Here's how the part is built. I have some questions about the finished solid (model axes, mm). Face numbers are marked on the shaded views. A direction names the side the tool comes from. Give positions to 0.01 mm unless a question says otherwise; leave off trailing zeros. Loops run counter-clockwise (first coordinate to the right, second up) from the corner with the lowest first, then second, coordinate; pieces in that order, holes last.
Q1. For the marked faces 1 and 2, which set-ups out of +Z, -Z, +X, -X, +Y, -Y let a thin tool reach every point of the face, with its end or its side?
Q2. I need wall thicknesses on probe 1 along Z at (x, y) = (6.25, 0.05); probe 2 along Z at (x, y) = (1, 0.6); probe 3 along Z at (x, y) = (3.5, 0.55). Which ranges of each line are inside material? Lowest first, please.
Q3. Suppose I cut it at A-A (x = 6). List the corners of the cut face in (y, z) for me.
Q4. I'm going to push a flat-ended pin straight in: P1, Ø1, axis at x = 3, z = 1, coming from the +Y side. Where does the tip first touch, or does it pass through?
```python
from build123d import *

# Parameters (mm, degrees)
RECPAT_COUNT = 2
RECPAT_ANGLE = 90


with BuildPart() as part:
    # Fillet1: read off the stored shape, not the designer's step
    # Fillet1 outline → Fillet1 (revolve)
    with BuildSketch(Plane.YX):
        with BuildLine():
            Line((1.25, 2.2), (1.25, 7.1))
            Line((1.25, 7.1), (0, 7.1))
            Line((0, 7.1), (0, 0))
            ThreePointArc((0, 0), (1.267435139, 0.206109099), (2.404255321, 0.803195916))
            ThreePointArc((2.404255321, 0.803195916), (2.474733878, 0.88781572), (2.5, 0.99500416))
            Line((2.5, 0.99500416), (2.5, 2.1))
            Line((2.5, 2.1), (1.35, 2.1))
            ThreePointArc((1.35, 2.1), (1.279289322, 2.129289322), (1.25, 2.2))
        make_face()
    revolve(axis=Axis((0, 0, 0), (1, 0, 0)))

    # Sketch3 → Recess section 0
    with BuildSketch(Plane(origin=(0, 0, 0), x_dir=(0, 0, -1), z_dir=(1, 0, 0))):
        with BuildLine():
            Line((0.37, -1.3), (-0.37, -1.3))
            Line((-0.37, -1.3), (-0.37, 1.3))
            Line((-0.37, 1.3), (0.37, 1.3))
            Line((0.37, 1.3), (0.37, -1.3))
        make_face()
    # Sketch4 → Recess section 1
    with BuildSketch(Plane(origin=(1.5, 0, 0), x_dir=(0, 0, -1), z_dir=(1, 0, 0))):
        with BuildLine():
            Line((0.37, -0.552127713), (-0.37, -0.552127713))
            Line((-0.37, -0.552127713), (-0.37, 0.552127713))
            Line((-0.37, 0.552127713), (0.37, 0.552127713))
            Line((0.37, 0.552127713), (0.37, -0.552127713))
        make_face()
    recess = loft(mode=Mode.SUBTRACT)

    # RecPat: Recess ×2 about axis
    recpat_axis = Axis((0, 0, 0), (1, 0, 0))
    for i in range(1, RECPAT_COUNT):
        add(recess.rotate(recpat_axis, i * RECPAT_ANGLE / (RECPAT_COUNT - 1)), mode=Mode.SUBTRACT)

    # RecCorSke → RecessCore (revolve, cut)
    with BuildSketch(Plane.XY, mode=Mode.PRIVATE) as recesscore_sk:
        Polygon((0, 0), (0, 0.660890218), (1.5, 0.556), (1.680655351, 0), align=None)
    revolve(recesscore_sk.sketch.rotate(Axis((-3.175, 0, 0), (1, 0, 0)), 90), axis=Axis((-3.175, 0, 0), (1, 0, 0)), mode=Mode.SUBTRACT)


solid = part.part
```
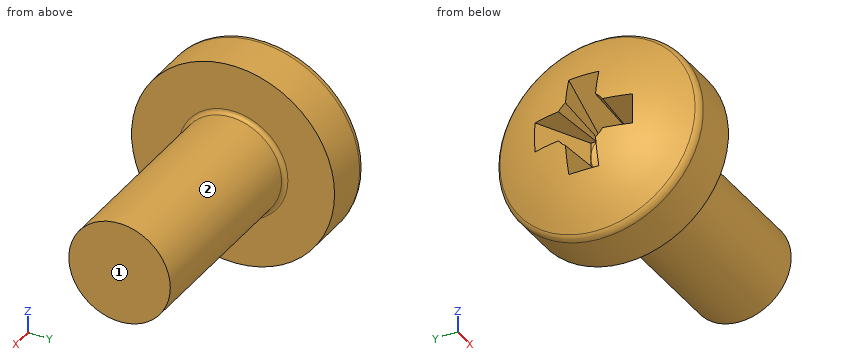
Solutions:
1. face 1: +Z, -Z, +X, +Y, -Y
1. face 2: +X
2. probe 1: z = -1.25 to 1.25
2. probe 2: z = -2.43 to -0.37, 0.37 to 2.43
2. probe 3: z = -1.12 to 1.12
3. outline: circle Ø2.5 at (0, 0)
4. P1: stops at y = 1.15
